from build123d import *

# Parameters (mm, degrees)
F0_R     = 1.55
F1_DEPTH = 2
F2_R     = 2.99999
F3_SIZE  = 0.2


# Not quite as in the source:
# - a fillet or chamfer is up to 0.001 mm smaller than in the source, because OpenCascade refuses the exact size


with BuildPart() as f1:
    # F0 (on Top) → F1 (new body)
    with BuildSketch(Plane.XY):
        with BuildLine():
            ThreePointArc((-15.25, 3), (-18.25, 0), (-15.25, -3))
            Line((-15.25, -3), (15.25, -3))
            ThreePointArc((15.25, -3), (18.25, 0), (15.25, 3))
            Line((15.25, 3), (4, 3))
            Line((4, 3), (-4, 3))
            Line((-4, 3), (-15.25, 3))
        make_face()
        with Locations((-15.25, 0)):
            Circle(F0_R, mode=Mode.SUBTRACT)
        with Locations((15.25, 0)):
            Circle(F0_R, mode=Mode.SUBTRACT)
        with BuildLine():
            Line((-4, 6), (-4, 3))
            Line((-4, 3), (4, 3))
            Line((4, 3), (4, 6))
            ThreePointArc((4, 6), (0, 10), (-4, 6))
        make_face()
        with Locations((0, 6)):
            Circle(F0_R, mode=Mode.SUBTRACT)
    extrude(amount=F1_DEPTH)

    # F2 (radius 3 in the source; OpenCascade refuses exactly that, so slightly less here)
    f2_edges = [f1.edges().sort_by_distance(p)[0] for p in [
        (4, 3, 1),
        (-4, 3, 1),
    ]]
    fillet(f2_edges, radius=F2_R)

    # F3
    f3_edges = [f1.edges().sort_by_distance(p)[0] for p in [
        (11.124995, 3, 0),
        (4.878677, 3.878677, 0),
        (18.25, 0, 0),
        (4, 5.999995, 0),
        (0, -3, 0),
        (0, 10, 0),
        (-18.25, 0, 0),
        (-4, 5.999995, 0),
        (-11.124995, 3, 0),
        (-4.878677, 3.878677, 0),
        (-16.8, 0, 0),
        (13.7, 0, 0),
        (-1.55, 6, 0),
    ]]
    chamfer(f3_edges, length=F3_SIZE)


solid = f1.part
Could you check a few things on this model? Use its own coordinates, in mm. A direction names the side the tool comes from. Coordinates: 2 decimals unless noted, no trailing zeros. Order: outer loops, then holes, each group sorted by start corner. A loop starts at its lowest first (then second) coordinate and runs counter-clockwise, first axis right, second up. Notation, with made-up numbers: (61.25, 12.5) - (96.25, 12.5) arc R31 cw to (96.25, 41.5) - close; hole circle Ø11 at (13.5, 43). An arc over 180 degrees is marked (long way). Answer in a Markdown table with one row per item. Add a question column.
(1) Will these pins go through, and if not, where does the flat tip stop? pin 1 (3 mm diameter, centred on x = 14, y = -0.5, fed in from +Z); pin 2 (3 mm diameter, centred on x = 0, y = 6, fed in from -Z).
(2) On a 3-axis mill with a long thin cutter (end or side, diameter ignored), from which of +Z, -Z, +X, -X, +Y, -Y can I reach the whole of each face in a straight line? I mean faces 4 (the face through (11, 3, 1)), 5 (the face through (-11, 3, 1)), 6 (the face through (0, 10, 1)). Say none if no direction works.
(3) I need wall thicknesses on L1, parallel to Y at x = 15.25, z = 1.15; L2, parallel to X at y = -0.5, z = 1.1; L3, parallel to Y at x = 0, z = 0.2. Which ranges of each line are inside material? Lowest first, please.
(4) If we mould it in two halves opening along X, with no side actions, what happens to faces 1 (the face through (-16.8, 0.07, 1.09)), 2 (the face through (-18.25, 0.07, 1.09)), 3 (the face through (0, 1, 0))? For each: released by +X, released by -X, zero draft, split by the parting line, or undercut.
(5) If we section it at C-C, the plane z = 1.5: State how many separate pieces and enclosed holes the cut face has, then the cut area to 3 significant figures.
(6) If we section it at D-D, the plane x = 8.5: Please give me the cut outline in (y, z).
(7) If we section it at A-A, the plane x = 0: Please give me the cut outline in (y, z).
(8) If we section it at B-B, the plane y = 0: Please give me the cut outline in (x, z).
Results are:
| question | item | result |
|---|---|---|
| 1 | pin 1 | stops at z = 2 |
| 1 | pin 2 | passes through |
| 2 | face 4 | +Z, -Z, +X, +Y |
| 2 | face 5 | +Z, -Z, -X, +Y |
| 2 | face 6 | +Z, -Z, +Y |
| 3 | L1 | y = -3 to -1.55, 1.55 to 3 |
| 3 | L2 | x = -18.21 to -16.72, -13.78 to 13.78, 16.72 to 18.21 |
| 3 | L3 | y = -3 to 4.45, 7.55 to 10 |
| 4 | face 1 | undercut |
| 4 | face 2 | released by -X |
| 4 | face 3 | zero draft |
| 5 | separate pieces | 1 |
| 5 | enclosed holes | 3 |
| 5 | area | 242 mm2 |
| 6 | outline | (-3, 0.2) - (-2.8, 0) - (2.8, 0) - (3, 0.2) - (3, 2) - (-3, 2) - close |
| 7 | outline | (-3, 0.2) - (-2.8, 0) - (4.25, 0) - (4.45, 0.2) - (4.45, 2) - (-3, 2) - close; (7.55, 0.2) - (7.75, 0) - (9.8, 0) - (10, 0.2) - (10, 2) - (7.55, 2) - close |
| 8 | outline | (-18.25, 0.2) - (-18.05, 0) - (-17, 0) - (-16.8, 0.2) - (-16.8, 2) - (-18.25, 2) - close; (-13.7, 0.2) - (-13.5, 0) - (13.5, 0) - (13.7, 0.2) - (13.7, 2) - (-13.7, 2) - close; (16.8, 0.2) - (17, 0) - (18.05, 0) - (18.25, 0.2) - (18.25, 2) - (16.8, 2) - close |
